```python
from build123d import *

# Parameters (mm, degrees)
SKETCH1_R               = 30.4
BOSS_EXTRUDE1_DEPTH     = 35
SKETCH4_W               = 4
SKETCH4_H               = 60.8
CUT_EXTRUDE1_DEPTH      = 30
LPATTERN1_COUNT         = 5
LPATTERN1_PITCH         = 6
MIRROR1_COPY_1_SKETCH_W = 4
MIRROR1_COPY_1_SKETCH_H = 60.8
MIRROR1_COPY_1_DEPTH    = 30
MIRROR1_COPY_2_SKETCH_W = 4
MIRROR1_COPY_2_SKETCH_H = 60.8
MIRROR1_COPY_2_DEPTH    = 30
MIRROR1_COPY_3_SKETCH_W = 4
MIRROR1_COPY_3_SKETCH_H = 60.8
MIRROR1_COPY_3_DEPTH    = 30
MIRROR1_COPY_4_SKETCH_W = 4
MIRROR1_COPY_4_SKETCH_H = 60.8
MIRROR1_COPY_4_DEPTH    = 30
MIRROR1_COPY_5_SKETCH_W = 4
MIRROR1_COPY_5_SKETCH_H = 60.8
MIRROR1_COPY_5_DEPTH    = 30
SKETCH9_W               = 4.4
SKETCH9_H               = 31.506189868
CUT_EXTRUDE2_DEPTH      = 30


with BuildPart() as part:
    # Sketch1 → Boss-Extrude1 (new body)
    with BuildSketch(Plane.XY):
        Circle(SKETCH1_R)
    extrude(amount=BOSS_EXTRUDE1_DEPTH)

    # Sketch4 → Cut-Extrude1 (cut)
    with BuildSketch(Plane(origin=(0, 0, 0), x_dir=(-1, 0, 0), z_dir=(0, 0, -1))):
        Rectangle(SKETCH4_W, SKETCH4_H)
    cut_extrude1 = extrude(amount=-CUT_EXTRUDE1_DEPTH, mode=Mode.SUBTRACT)

    # LPattern1: Cut-Extrude1 ×5
    with Locations(*[(i * LPATTERN1_PITCH, 0, 0) for i in range(1, LPATTERN1_COUNT)]):
        add(cut_extrude1, mode=Mode.SUBTRACT)

    # Mirror1 copy 1 sketch → Mirror1 copy 1 (cut)
    with BuildSketch(Plane(origin=(-6, 0, 0), x_dir=(1, 0, 0), z_dir=(0, 0, -1))):
        Rectangle(MIRROR1_COPY_1_SKETCH_W, MIRROR1_COPY_1_SKETCH_H)
    extrude(amount=-MIRROR1_COPY_1_DEPTH, mode=Mode.SUBTRACT)

    # Mirror1 copy 2 sketch → Mirror1 copy 2 (cut)
    with BuildSketch(Plane(origin=(-12, 0, 0), x_dir=(1, 0, 0), z_dir=(0, 0, -1))):
        Rectangle(MIRROR1_COPY_2_SKETCH_W, MIRROR1_COPY_2_SKETCH_H)
    extrude(amount=-MIRROR1_COPY_2_DEPTH, mode=Mode.SUBTRACT)

    # Mirror1 copy 3 sketch → Mirror1 copy 3 (cut)
    with BuildSketch(Plane(origin=(-18, 0, 0), x_dir=(1, 0, 0), z_dir=(0, 0, -1))):
        Rectangle(MIRROR1_COPY_3_SKETCH_W, MIRROR1_COPY_3_SKETCH_H)
    extrude(amount=-MIRROR1_COPY_3_DEPTH, mode=Mode.SUBTRACT)

    # Mirror1 copy 4 sketch → Mirror1 copy 4 (cut)
    with BuildSketch(Plane(origin=(-24, 0, 0), x_dir=(1, 0, 0), z_dir=(0, 0, -1))):
        Rectangle(MIRROR1_COPY_4_SKETCH_W, MIRROR1_COPY_4_SKETCH_H)
    extrude(amount=-MIRROR1_COPY_4_DEPTH, mode=Mode.SUBTRACT)

    # Mirror1 copy 5 sketch → Mirror1 copy 5 (cut)
    with BuildSketch(Plane(origin=(0, 0, 0), x_dir=(1, 0, 0), z_dir=(0, 0, -1))):
        Rectangle(MIRROR1_COPY_5_SKETCH_W, MIRROR1_COPY_5_SKETCH_H)
    extrude(amount=-MIRROR1_COPY_5_DEPTH, mode=Mode.SUBTRACT)

    # Sketch9 → Cut-Extrude2 (cut)
    with BuildSketch(Plane(origin=(0, 0, 0), x_dir=(-1, 0, 0), z_dir=(0, 0, -1))):
        with Locations((-28.2, 0)):
            Rectangle(SKETCH9_W, SKETCH9_H)
        with Locations((28.2, 0)):
            Rectangle(SKETCH9_W, SKETCH9_H)
    extrude(amount=-CUT_EXTRUDE2_DEPTH, mode=Mode.SUBTRACT)

    # Sketch14 → CBORE for #2 Binding Head Machine Screw2 (revolve, cut)
    with BuildSketch(Plane(origin=(26.4, 0, 30), x_dir=(0, 1, 0), z_dir=(1, 0, 0))):
        Polygon((0, 0), (0, 5.732569267), (1.2192, 5), (1.2192, 1.27), (2.77876, 1.27), (2.77876, 0), align=None)
    cbore_for_2_binding_head_machine_screw2 = revolve(axis=Axis((26.4, 0, 23.65), (0, 0, 1)), mode=Mode.SUBTRACT)

    # Mirror2: CBORE for #2 Binding Head Machine Screw2 across plane
    add(cbore_for_2_binding_head_machine_screw2.mirror(Plane(origin=(0, 0, 0), x_dir=(0, 0, 1), z_dir=(1, 0, 0))), mode=Mode.SUBTRACT)


solid = part.part
```
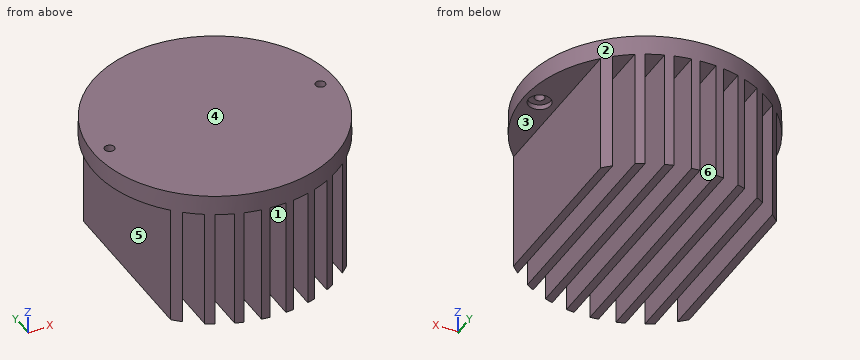
Here's how the part is built. I have some questions about the finished solid (model axes, mm). Face numbers are marked on the shaded views. A direction names the side the tool comes from. Coordinates: 2 decimals unless noted, no trailing zeros. Loops run counter-clockwise (first coordinate to the right, second up) from the corner with the lowest first, then second, coordinate; pieces in that order, holes last. Notation, with made-up numbers: (49, -35) - (70, -35) arc R27 ccw to (70, 1) - close; hole circle Ø8 at (50, 11). An arc over 180 degrees is marked (long way). Answer as CSV lines item,"result".
Q1. For pin 1 (5 mm diameter, centred on y = 14.5, z = 24.5, fed in from -X); pin 2 (1.2 mm diameter, centred on x = 19, y = 1.5, fed in from -Z); pin 3 (1 mm diameter, centred on x = -2.5, z = 8, fed in from -Y), each with a flat end and sliding along its axis, tell me the tip position at first contact or that it passes through.
Response:
pin 1,"x = -22"
pin 2,"z = 30"
pin 3,"y = -30.33"
Q2. If we section it at D-D, the plane y = -24: Write out the boundary of the cut face in (x, z).
Response:
outline,"(-18.66, 30) - (-16, 30) - (-16, 0) - (-14, 0) - (-14, 30) - (-10, 30) - (-10, 0) - (-8, 0) - (-8, 30) - (-4, 30) - (-4, 0) - (-2, 0) - (-2, 30) - (2, 30) - (2, 0) - (4, 0) - (4, 30) - (8, 30) - (8, 0) - (10, 0) - (10, 30) - (14, 30) - (14, 0) - (16, 0) - (16, 30) - (18.66, 30) - (18.66, 35) - (-18.66, 35) - close"
Q3. If we section it at A-A, the plane z = 20: Give the number of separate pieces and of enclosed holes in the cut face, and give its area (3 significant figures).
Response:
separate pieces,"8"
enclosed holes,"0"
area,"861 mm2"
Q4. If we section it at B-B, the plane x = -26.4: Write out the boundary of the cut face in (y, z).
Response:
outline,"(-15.07, 30) - (-2.78, 30) - (-2.78, 31.27) - (-1.22, 31.27) - (-1.22, 35) - (-15.07, 35) - close; (1.22, 31.27) - (2.78, 31.27) - (2.78, 30) - (15.07, 30) - (15.07, 35) - (1.22, 35) - close"
Q5. For the marked faces 1, 2 and 3, which set-ups out of +Z, -Z, +X, -X, +Y, -Y let a thin tool reach every point of the face, with its end or its side?
Response:
face 1,"-Z, +Y, -Y"
face 2,"+Z, -Z"
face 3,"-Z, +X, +Y, -Y"
Q6. If I drill on L1, parallel to X at y = 0, z = 32.45; L2, parallel to X at y = 0, z = 30.95; L3, parallel to X at y = 23, z = 23, over which ranges is the centre line in solid material (lowest first)? Write a range as [from, to].
Response:
L1,"[-30.4, -27.62], [-25.18, 25.18], [27.62, 30.4]"
L2,"[-30.4, -29.18], [-23.62, 23.62], [29.18, 30.4]"
L3,"[-16, -14], [-10, -8], [-4, -2], [2, 4], [8, 10], [14, 16]"
Q7. We'd pull the mould along X, two halves only. Please class the marked faces 4, 5 and 6: pulls with the +X half, pulls with the -X half, needs draft (parallel to the pull), parting line crosses it, or undercut.
Response:
face 4,"needs draft"
face 5,"pulls with the -X half"
face 6,"undercut"
